from build123d import *

# Parameters (mm, degrees)
BOSS_EXTRU_1_DEPTH           = 75
ENL_V_MAT_EXTRU_9_DEPTH      = 1
ENL_V_MAT_EXTRU_9_DEPTH_BACK = 3


with BuildPart() as part:
    # Esquisse2 → Boss.-Extru.1 (new body)
    with BuildSketch(Plane(origin=(0, 0, 0), x_dir=(1, 0, 0), z_dir=(0, 1, 0))):
        Polygon((0, 0), (0, 8), (10, 8), (10, 6), (2, 6), (2, 0), align=None)
    extrude(amount=BOSS_EXTRU_1_DEPTH)

    # Esquisse3 → Enlèv. mat.-Extru.9 (cut, two sides: drawn at the far end of the back side and taken through both)
    with BuildSketch(Plane(origin=(2, 0, 0), x_dir=(0, 0, -1), z_dir=(1, 0, 0)).offset(-ENL_V_MAT_EXTRU_9_DEPTH_BACK)):
        with BuildLine():
            Line((6, 38.672788966), (6, 35.672788966))
            Line((6, 35.672788966), (5, 35.672788966))
            ThreePointArc((5, 35.672788966), (3.5, 37.172788966), (5, 38.672788966))
            Line((5, 38.672788966), (6, 38.672788966))
        make_face()
        with BuildLine():
            Line((6, 63.672788966), (5, 63.672788966))
            ThreePointArc((5, 63.672788966), (3.5, 65.172788966), (5, 66.672788966))
            Line((5, 66.672788966), (6, 66.672788966))
            Line((6, 66.672788966), (6, 63.672788966))
        make_face()
        with BuildLine():
            Line((6, 7.672788966), (5, 7.672788966))
            ThreePointArc((5, 7.672788966), (3.5, 9.172788966), (5, 10.672788966))
            Line((5, 10.672788966), (6, 10.672788966))
            Line((6, 10.672788966), (6, 7.672788966))
        make_face()
    extrude(amount=ENL_V_MAT_EXTRU_9_DEPTH + ENL_V_MAT_EXTRU_9_DEPTH_BACK, mode=Mode.SUBTRACT)


solid = part.part
Part model, mm, in its own coordinate system. A direction names the side the tool comes from. Coordinates: 2 decimals unless noted, no trailing zeros. Loops run counter-clockwise (first coordinate to the right, second up) from the corner with the lowest first, then second, coordinate; pieces in that order, holes last. Notation, with made-up numbers: M 26,10 L 73,10 A36 ccw 73,49 Z; hole C 76.5,52 d11. An arc over 180 degrees is marked long. Use a Markdown table: item, result. Add a question column.
Q1. Cut at B-B (y = 37). Write the cut outline in (x, z), and give its area (3 significant figures).
Q2. Probe L1, parallel to Y at x = 1.5, z = -5.5; L2, parallel to Y at x = 1, z = -4; L3, parallel to X at y = 44.5, z = -5.5. List the from-to ranges inside material, lowest first.
Q3. Cut at A-A (x = 1). Write the cut outline in (y, z).
Q4. Cut at D-D (z = -2.5). Write the cut outline in (x, y).
Q5. Pin check, flat tips, straight feed: P1, Ø4, axis at x = 5, y = 52.5, coming from the +Z side; P2, Ø3, axis at y = 45.5, z = -3.5, coming from the +X side; P3, Ø3, axis at x = 4.5, z = -3.5, coming from the -Y side. Stop position of each tip, or through.
Q6. Cut at C-C (y = 48.5). Write the cut outline in (x, z).
Q7. Which spindle directions (+Z, -Z, +X, -X, +Y, -Y) get a long thin tool onto all of the face, cutting with end or side? Do faces 5 (the flat face through (2, 37, -3)), 6 (the flat face through (3, 0, -7)), 7 (the cylindrical face through (1, 37.1, -3.5)). Say none if no direction does.
Q8. Mould opens along Z. For faces 1 (the cylindrical face through (1, 9.1, -3.5)), 2 (the flat face through (1, 37, 0)), 3 (the flat face through (5, 37, -8)), 4 (the cylindrical face through (1, 65.1, -3.5)) say: +Z half, -Z half, draft (parallel to the pull), parting line (faces both ways), or undercut.
Worked out:
| question | item | result |
|---|---|---|
| 1 | outline | M 0,-8 L 10,-8 L 10,-6 L 0,-6 Z; M 0,-3.51 L 2,-3.51 L 2,0 L 0,0 Z |
| 1 | area | 27.0 mm2 |
| 2 | L1 | y = 0 to 7.67, 10.67 to 35.67, 38.67 to 63.67, 66.67 to 75 |
| 2 | L2 | y = 0 to 8.05, 10.29 to 36.05, 38.29 to 64.05, 66.29 to 75 |
| 2 | L3 | x = 0 to 2 |
| 3 | outline | M 0,-8 L 75,-8 L 75,0 L 0,0 Z; hole M 7.67,-6 L 10.67,-6 L 10.67,-5 A1.5 ccw 7.67,-5 Z; hole M 35.67,-6 L 38.67,-6 L 38.67,-5 A1.5 ccw 35.67,-5 Z; hole M 63.67,-6 L 66.67,-6 L 66.67,-5 A1.5 ccw 63.67,-5 Z |
| 4 | outline | M 0,0 L 2,0 L 2,75 L 0,75 Z |
| 5 | P1 | stops at z = -6 |
| 5 | P2 | stops at x = 2 |
| 5 | P3 | passes through |
| 6 | outline | M 0,-8 L 10,-8 L 10,-6 L 2,-6 L 2,0 L 0,0 Z |
| 7 | face 5 | +Z, +X, +Y, -Y |
| 7 | face 6 | +Z, -Z, +X, -X, -Y |
| 7 | face 7 | +X, -X |
| 8 | face 1 | undercut |
| 8 | face 2 | +Z half |
| 8 | face 3 | -Z half |
| 8 | face 4 | undercut |
